Here's the drawing with two shaded views (mm, measured from the low corner). I have some questions. A direction names the side the tool comes from. Round coordinates to 2 decimals unless told otherwise and drop trailing zeros. Write each loop counter-clockwise with the first axis right and the second up, starting at its lowest first coordinate (ties: lowest second). Pieces come first, ordered by that corner, then holes. Notation, with made-up numbers: M 87,-39.75 L 112,-39.75 A8 ccw 112,-26.75 Z; hole C 50,73 d1. An arc over 180 degrees is marked long. Use one line per item in the form item = value. Start each with the question number.
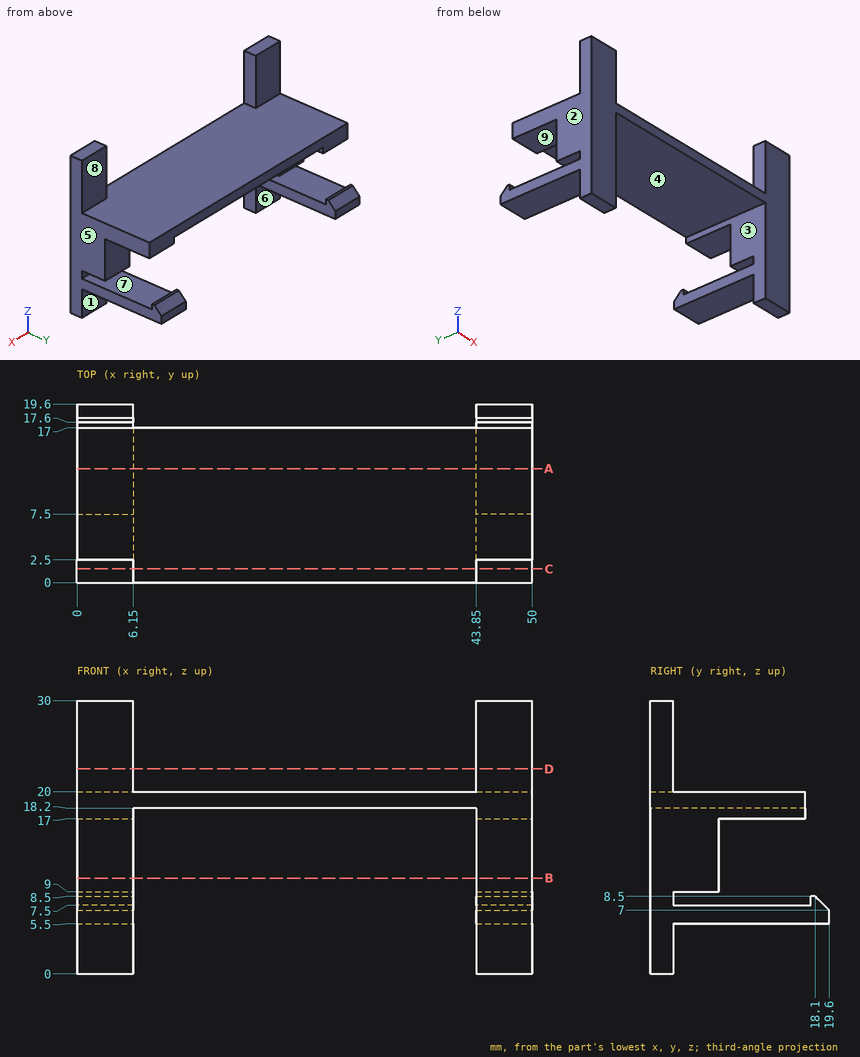
1. Please list where these lines run through material, in increasing order: line 1 along X through (y, z) = (1.75, 15.75); line 2 along Z through (x, y) = (36.5, 7); line 3 along Z through (x, y) = (3, 17.5).
2. Will these pins go through, and if not, where does the flat tip stop? pin 1 (3 mm diameter, centred on x = 3, y = 14.5, fed in from -Z); pin 2 (1.8 mm diameter, centred on x = 4.5, y = 6.5, fed in from +Z); pin 3 (4.5 mm diameter, centred on x = 4, z = 2.5, fed in from +Y).
3. If we section it at A-A (y = 12.5): List the corners of the cut face in (x, z) for me.
4. If we section it at C-C (y = 1.5): List the corners of the cut face in (x, z) for me.
5. If we mould it in two halves opening along X, with no side actions, what happens to the marked faces 1, 2, 3 and 4? For each: pulls with the +X half, pulls with the -X half, needs draft (parallel to the pull), parting line crosses it, or undercut.
6. Which directions (+Z, -Z, +X, -X, +Y, -Y) give clear straight access to the entire face, cutting with the end or side of a thin tool? Please do the marked faces 5, 6, 7, 8 and 9.
7. If we section it at B-B (z = 10.5): List the corners of the cut face in (x, y) for me.
8. If we section it at D-D (z = 22.5): List the corners of the cut face in (x, y) for me, and give its area (4 significant figures).
Model answer:
q1.line_1 = 0 to 6.15, 43.85 to 50
q1.line_2 = 18.2 to 20
q1.line_3 = 5.5 to 7.5
q2.pin_1 = 5.5
q2.pin_2 = 20
q2.pin_3 = 2.5
q3.outline = M 0,5.5 L 6.15,5.5 L 6.15,7.5 L 0,7.5 Z; M 0,17 L 6.15,17 L 6.15,18.2 L 43.85,18.2 L 43.85,17 L 50,17 L 50,20 L 0,20 Z; M 43.85,5.5 L 50,5.5 L 50,7.5 L 43.85,7.5 Z
q4.outline = M 0,0 L 6.15,0 L 6.15,18.2 L 43.85,18.2 L 43.85,0 L 50,0 L 50,30 L 43.85,30 L 43.85,20 L 6.15,20 L 6.15,30 L 0,30 Z
q5.face_1 = needs draft
q5.face_2 = pulls with the -X half
q5.face_3 = undercut
q5.face_4 = undercut
q6.face_5 = +Z, -Z, +X, +Y, -Y
q6.face_6 = -Z, +X, -X, +Y
q6.face_7 = +X, -X
q6.face_8 = +Z, +X, -X, +Y
q6.face_9 = +X, -X, +Y
q7.outline = M 0,0 L 6.15,0 L 6.15,7.5 L 0,7.5 Z; M 43.85,0 L 50,0 L 50,7.5 L 43.85,7.5 Z
q8.outline = M 0,0 L 6.15,0 L 6.15,2.5 L 0,2.5 Z; M 43.85,0 L 50,0 L 50,2.5 L 43.85,2.5 Z
q8.area = 30.75 mm2
